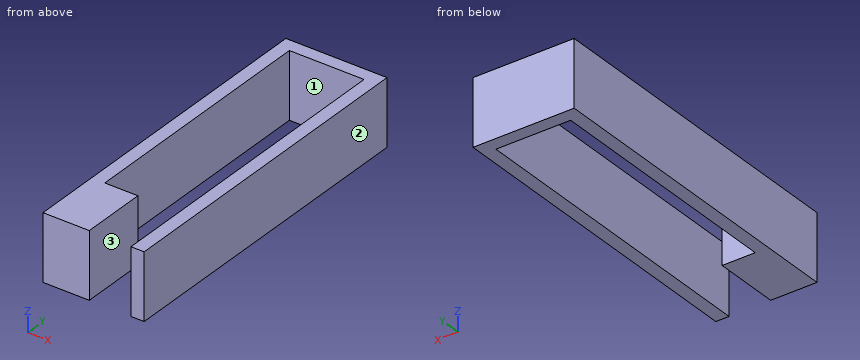
```python
from build123d import *

# Parameters (mm, degrees)
F0_W     = 6.35
F0_H     = 12.7
F0_W_2   = 14.351
F0_H_2   = 2.54
F1_DEPTH = 12.7


with BuildPart() as f1:
    # F0 (on Top) → F1 (new body)
    with BuildSketch(Plane.XY):
        with Locations((-12.446, -25.4)):
            Rectangle(F0_W, F0_H)
        Polygon((-15.621, -19.05), (-15.621, 29.21), (-15.621, 31.75), (-18.161, 31.75), (-18.161, -31.75), (-15.621, -31.75), align=None)
        with Locations((-8.4455, 30.48)):
            Rectangle(F0_W_2, F0_H_2)
        Polygon((-1.27, -31.75), (1.27, -31.75), (1.27, 31.75), (-1.27, 31.75), (-1.27, 29.21), align=None)
    extrude(amount=F1_DEPTH)


solid = f1.part
```
CAD build for the part. Positions are in the model's coordinates, mm. Face numbers are marked on the shaded views. A direction names the side the tool comes from. Give positions to 0.01 mm unless a question says otherwise; leave off trailing zeros. Order: outer loops, then holes, each group sorted by start corner. A loop starts at its lowest first (then second) coordinate and runs counter-clockwise, first axis right, second up. Notation, with made-up numbers: M 21,16.5 L 37,16.5 A22 cw 37,48.5 Z; hole C 51,69 d2. An arc over 180 degrees is marked long. Put each result on its own line as item: value. Start each with the question number.
(1) Saw through at D-D, the plane x = -6.5. Write the cut outline in (y, z), then the cut area to 3 significant figures.
(2) Saw through at C-C, the plane z = 3.25. Write the cut outline in (x, y).
(3) Saw through at A-A, the plane y = -21.5. Write the cut outline in (x, z).
(4) Flat gauge pin, fed straight in: pin 1 Ø4 at (x, z) = (-7.5, 9) entering from -Y. Where does the tip first touch, or does it go through?
(5) Drill centre lines: line 1 along X through (y, z) = (23, 5); line 2 along X through (y, z) = (-24, 4.75); line 3 along Y through (x, z) = (-10.25, 9.5). Where is each one in solid material? Low to high.
(6) Which spindle directions (+Z, -Z, +X, -X, +Y, -Y) get a long thin tool onto all of the face, cutting with end or side? Do the marked faces 1, 2 and 3. Say none if no direction does.
(7) Saw through at B-B, the plane x = -11.5. Write the cut outline in (y, z), then the cut area to 3 significant figures.
Check result:
1. outline: M 29.21,0 L 31.75,0 L 31.75,12.7 L 29.21,12.7 Z
1. area: 32.3 mm2
2. outline: M -18.16,-31.75 L -9.27,-31.75 L -9.27,-19.05 L -15.62,-19.05 L -15.62,29.21 L -1.27,29.21 L -1.27,-31.75 L 1.27,-31.75 L 1.27,31.75 L -18.16,31.75 Z
3. outline: M -18.16,0 L -9.27,0 L -9.27,12.7 L -18.16,12.7 Z; M -1.27,0 L 1.27,0 L 1.27,12.7 L -1.27,12.7 Z
4. pin 1: stops at y = -31.75
5. line 1: x = -18.16 to -15.62, -1.27 to 1.27
5. line 2: x = -18.16 to -9.27, -1.27 to 1.27
5. line 3: y = -31.75 to -19.05, 29.21 to 31.75
6. face 1: +Z, -Z
6. face 2: +Z, -Z, +X, +Y, -Y
6. face 3: +Z, -Z, -Y
7. outline: M -31.75,0 L -19.05,0 L -19.05,12.7 L -31.75,12.7 Z; M 29.21,0 L 31.75,0 L 31.75,12.7 L 29.21,12.7 Z
7. area: 194 mm2
